from build123d import *

# Parameters (mm, degrees)
SKETCH1_R           = 34.671
BOSS_EXTRUDE1_DEPTH = 25.4
SKETCH2_R           = 25.4
CUT_EXTRUDE1_DEPTH  = 20.066
SKETCH4_R           = 4.826
BOSS_EXTRUDE2_DEPTH = 20.066
SKETCH5_R           = 2.667
CUT_EXTRUDE2_DEPTH  = 20.066
CUT_EXTRUDE3_DEPTH  = 53.979249126


with BuildPart() as part:
    # Sketch1 → Boss-Extrude1 (new body)
    with BuildSketch(Plane(origin=(0, 0, 0), x_dir=(1, 0, 0), z_dir=(0, 1, 0))):
        with Locations(Location((0, 0, 0), (0, 0, 270))):
            Circle(SKETCH1_R)
    extrude(amount=BOSS_EXTRUDE1_DEPTH)

    # Sketch2 → Cut-Extrude1 (cut)
    with BuildSketch(Plane(origin=(0, 25.4, 0), x_dir=(1, 0, 0), z_dir=(0, 1, 0))):
        with Locations(Location((0, 0, 0), (0, 0, 270))):
            Circle(SKETCH2_R)
    extrude(amount=-CUT_EXTRUDE1_DEPTH, mode=Mode.SUBTRACT)

    # Sketch4 → Boss-Extrude2 (add)
    with BuildSketch(Plane(origin=(0, 5.334, 0), x_dir=(1, 0, 0), z_dir=(0, 1, 0))):
        with Locations(Location((0, 0, 0), (0, 0, 270))):
            Circle(SKETCH4_R)
    extrude(amount=BOSS_EXTRUDE2_DEPTH)

    # Sketch5 → Cut-Extrude2 (cut)
    with BuildSketch(Plane(origin=(0, 25.4, 0), x_dir=(1, 0, 0), z_dir=(0, 1, 0))):
        with Locations(Location((0, 0, 0), (0, 0, 270))):
            Circle(SKETCH5_R)
    extrude(amount=-CUT_EXTRUDE2_DEPTH, mode=Mode.SUBTRACT)

    # Sketch6 → Cut-Extrude3 (cut, through all)
    with BuildSketch(Plane(origin=(0, 5.334, 0), x_dir=(1, 0, 0), z_dir=(0, 1, 0))):
        with BuildLine():
            ThreePointArc((-20.672131698, 14.758826886), (-22.029333921, 12.643909483), (-23.170911404, 10.405232564))
            Line((-23.170911404, 10.405232564), (-4.402473167, 1.976994187))
            ThreePointArc((-4.402473167, 1.976994187), (-4.185573445, 2.402342802), (-3.927705023, 2.804177108))
            Line((-3.927705023, 2.804177108), (-20.672131698, 14.758826886))
        make_face()
        with BuildLine():
            Line((-15.913974648, 19.796600993), (-3.023655183, 3.761354189))
            ThreePointArc((-3.023655183, 3.761354189), (-2.626023591, 4.048984577), (-2.201236583, 4.294744871))
            Line((-2.201236583, 4.294744871), (-11.585455702, 22.603920372))
            ThreePointArc((-11.585455702, 22.603920372), (-13.821176792, 21.31044514), (-15.913974648, 19.796600993))
        make_face()
        with BuildLine():
            Line((-7.956987324, 24.121491511), (-1.511827592, 4.583083387))
            ThreePointArc((-1.511827592, 4.583083387), (-1.13757061, 4.690011632), (-0.755913796, 4.766431614))
            Line((-0.755913796, 4.766431614), (-3.978493662, 25.08648218))
            ThreePointArc((-3.978493662, 25.08648218), (-5.987213738, 24.684271747), (-7.956987324, 24.121491511))
        make_face()
        with BuildLine():
            Line((0, 25.4), (0, 4.826))
            ThreePointArc((0, 4.826), (0.496889313, 4.800351759), (0.988497094, 4.723679656))
            Line((0.988497094, 4.723679656), (5.202616282, 24.861471876))
            ThreePointArc((5.202616282, 24.861471876), (2.61520691, 25.265009258), (0, 25.4))
        make_face()
        with BuildLine():
            Line((10.405232564, 23.170911404), (1.976994187, 4.402473167))
            ThreePointArc((1.976994187, 4.402473167), (2.402342802, 4.185573445), (2.804177108, 3.927705023))
            Line((2.804177108, 3.927705023), (14.758826886, 20.672131698))
            ThreePointArc((14.758826886, 20.672131698), (12.643909483, 22.029333921), (10.405232564, 23.170911404))
        make_face()
        with BuildLine():
            Line((19.240686042, 16.581797268), (3.655730348, 3.150541481))
            ThreePointArc((3.655730348, 3.150541481), (3.93490279, 2.794068008), (4.179438599, 2.413))
            Line((4.179438599, 2.413), (21.997045256, 12.7))
            ThreePointArc((21.997045256, 12.7), (20.710014683, 14.705621097), (19.240686042, 16.581797268))
        make_face()
        with BuildLine():
            Line((23.786716405, 8.90798084), (4.519476117, 1.69251636))
            ThreePointArc((4.519476117, 1.69251636), (4.654621925, 1.274664949), (4.751223326, 0.84625818))
            Line((4.751223326, 0.84625818), (25.006438558, 4.45399042))
            ThreePointArc((25.006438558, 4.45399042), (24.498010133, 6.708762891), (23.786716405, 8.90798084))
        make_face()
        with BuildLine():
            Line((25.4, 0), (4.826, 0))
            ThreePointArc((4.826, 0), (4.800351759, -0.496889313), (4.723679656, -0.988497094))
            Line((4.723679656, -0.988497094), (24.861471876, -5.202616282))
            ThreePointArc((24.861471876, -5.202616282), (25.265009258, -2.61520691), (25.4, 0))
        make_face()
        with BuildLine():
            Line((23.170911404, -10.405232564), (4.402473167, -1.976994187))
            ThreePointArc((4.402473167, -1.976994187), (4.115324299, -2.520789939), (3.761354189, -3.023655183))
            Line((3.761354189, -3.023655183), (19.796600993, -15.913974648))
            ThreePointArc((19.796600993, -15.913974648), (21.659601572, -13.267315469), (23.170911404, -10.405232564))
        make_face()
        with BuildLine():
            Line((15.913974648, -19.796600993), (3.023655183, -3.761354189))
            ThreePointArc((3.023655183, -3.761354189), (2.626023591, -4.048984577), (2.201236583, -4.294744871))
            Line((2.201236583, -4.294744871), (11.585455702, -22.603920372))
            ThreePointArc((11.585455702, -22.603920372), (13.821176792, -21.31044514), (15.913974648, -19.796600993))
        make_face()
        with BuildLine():
            Line((7.956987324, -24.121491511), (1.511827592, -4.583083387))
            ThreePointArc((1.511827592, -4.583083387), (1.00639234, -4.719899412), (0.489109394, -4.801150695))
            Line((0.489109394, -4.801150695), (2.574259969, -25.269214187))
            ThreePointArc((2.574259969, -25.269214187), (5.296801792, -24.841575851), (7.956987324, -24.121491511))
        make_face()
        with BuildLine():
            Line((0, -25.4), (0, -4.826))
            ThreePointArc((0, -4.826), (-0.496889313, -4.800351759), (-0.988497094, -4.723679656))
            Line((-0.988497094, -4.723679656), (-5.202616282, -24.861471876))
            ThreePointArc((-5.202616282, -24.861471876), (-2.61520691, -25.265009258), (0, -25.4))
        make_face()
        with BuildLine():
            Line((-10.405232564, -23.170911404), (-1.976994187, -4.402473167))
            ThreePointArc((-1.976994187, -4.402473167), (-2.520789939, -4.115324299), (-3.023655183, -3.761354189))
            Line((-3.023655183, -3.761354189), (-15.913974648, -19.796600993))
            ThreePointArc((-15.913974648, -19.796600993), (-13.267315469, -21.659601572), (-10.405232564, -23.170911404))
        make_face()
        with BuildLine():
            Line((-19.240686042, -16.581797268), (-3.655730348, -3.150541481))
            ThreePointArc((-3.655730348, -3.150541481), (-3.93490279, -2.794068008), (-4.179438599, -2.413))
            Line((-4.179438599, -2.413), (-21.997045256, -12.7))
            ThreePointArc((-21.997045256, -12.7), (-20.710014683, -14.705621097), (-19.240686042, -16.581797268))
        make_face()
        with BuildLine():
            Line((-4.751223326, -0.84625818), (-25.006438558, -4.45399042))
            ThreePointArc((-25.006438558, -4.45399042), (-24.498010133, -6.708762891), (-23.786716405, -8.90798084))
            Line((-23.786716405, -8.90798084), (-4.519476117, -1.69251636))
            ThreePointArc((-4.519476117, -1.69251636), (-4.654621925, -1.274664949), (-4.751223326, -0.84625818))
        make_face()
        with BuildLine():
            ThreePointArc((-24.861471876, 5.202616282), (-25.265009258, 2.61520691), (-25.4, 0))
            Line((-25.4, 0), (-4.826, 0))
            ThreePointArc((-4.826, 0), (-4.800351759, 0.496889313), (-4.723679656, 0.988497094))
            Line((-4.723679656, 0.988497094), (-24.861471876, 5.202616282))
        make_face()
    extrude(amount=-CUT_EXTRUDE3_DEPTH, mode=Mode.SUBTRACT)


solid = part.part
Input: part model. Units: mm. Frame: model coordinates. A direction names the side the tool comes from. Round coordinates to 2 decimals unless told otherwise and drop trailing zeros. Write each loop counter-clockwise with the first axis right and the second up, starting at its lowest first coordinate (ties: lowest second). Pieces come first, ordered by that corner, then holes.
1) Cut plane D-D (z = -28). Return the cut outline in (x, y).
2) Cut plane B-B (x = -30). Return the cut outline in (y, z), then the cut area to 3 significant figures.
3) Contact query for flat-ended pins moving along their axis: P1, Ø2.5, axis at x = -0.5, z = -1, coming from the +Y side; P2, Ø8, axis at y = 3, z = -4, coming from the +X side; P3, Ø12, axis at y = 13, z = 16.5, coming from the +X side. Output: stop coordinate, or through.
4) Cut plane A-A (y = 12.5). Return the cut outline in (x, z).
5) Cut plane C-C (x = -7). Count the separate pieces of the cut face and the enclosed holes in it, then the cut area to 3 significant figures.
6) Draft query along Z for faces 1 (the flat face through (1.517, 2.704, 14.892)), 2 (the flat face through (-2, 25.4, 2)). Return one class per face: pulls with the +Z half, pulls with the -Z half, needs draft (parallel to the pull), parting line crosses it, or undercut.
7) Reachability of faces 3 (the flat face through (0, 0, 0)), 4 (the flat face through (11.67, 2.7, 9.38)), 5 (the flat face through (-2, 5.334, -18)) from +Z, -Z, +X, -X, +Y, -Y: full face, straight path, thin tool, end or side. Return the list, or none.
8) Ray query, L1, parallel to X at y = 17.75, z = 0; L2, parallel to Z at x = -4, y = 19.75; L3, parallel to X at y = 5.25, z = 17. Return the intervals inside material, ascending.
Geometry says:
1. outline: (-20.45, 0) - (20.45, 0) - (20.45, 25.4) - (-20.45, 25.4) - close
2. outline: (0, -17.38) - (25.4, -17.38) - (25.4, 17.38) - (0, 17.38) - close
2. area: 883 mm2
3. P1: stops at y = 5.33
3. P2: stops at x = 34.67
3. P3: stops at x = 33.04
4. outline: circle Ø69.34 at (0, 0); circle Ø9.65 at (0, 0); hole circle Ø50.8 at (0, 0); hole circle Ø5.33 at (0, 0)
5. separate pieces: 8
5. enclosed holes: 0
5. area: 629 mm2
6. face 1: undercut
6. face 2: needs draft
7. face 3: +Z, -Z, +X, -X, -Y
7. face 4: +Y, -Y
7. face 5: +Y
8. L1: x = -34.67 to -25.4, -4.83 to -2.67, 2.67 to 4.83, 25.4 to 34.67
8. L2: z = -34.44 to -25.08, -2.7 to 2.7, 25.08 to 34.44
8. L3: x = -30.22 to -13.67, -7.63 to -3.56, 0 to 1.73, 5.61 to 8.71, 13.67 to 30.22
